Design review of the part built by this model. Coordinates are the model's own, in mm. A direction names the side the tool comes from. Coordinates: 2 decimals unless noted, no trailing zeros. Write each loop counter-clockwise with the first axis right and the second up, starting at its lowest first coordinate (ties: lowest second). Pieces come first, ordered by that corner, then holes. Notation, with made-up numbers: M -26,47 L 14,47 A15 cw 14,65 Z; hole C -9,-20.5 d8. An arc over 180 degrees is marked long. One line per question, with ' | ' between items.
from build123d import *

# Parameters (mm, degrees)
F0_W     = 50
F0_H     = 32
F0_R     = 1.25
F0_W_2   = 15
F0_H_2   = 4.5
F1_DEPTH = 10
F2_SIZE  = 5


with BuildPart() as f1:
    # F0 (on Top) → F1 (new body)
    with BuildSketch(Plane.XY):
        with Locations((25, 16)):
            Rectangle(F0_W, F0_H)
        with Locations((20, 4.85)):
            Circle(F0_R, mode=Mode.SUBTRACT)
        with Locations((30, 4.85)):
            Circle(F0_R, mode=Mode.SUBTRACT)
        with Locations((10, 16)):
            Rectangle(F0_W_2, F0_H_2, mode=Mode.SUBTRACT)
        with Locations((20, 27.15)):
            Circle(F0_R, mode=Mode.SUBTRACT)
        with Locations((40, 16)):
            Rectangle(F0_W_2, F0_H_2, mode=Mode.SUBTRACT)
        with Locations((30, 27.15)):
            Circle(F0_R, mode=Mode.SUBTRACT)
    extrude(amount=F1_DEPTH)

    # F2
    f2_edges = [f1.edges().sort_by_distance(p)[0] for p in [
        (0, 0, 5),
        (50, 0, 5),
        (50, 32, 5),
        (0, 32, 5),
    ]]
    chamfer(f2_edges, length=F2_SIZE)


solid = f1.part
1. Take a section at B-B (x = 30). Write out the cut boundary in (y, z).
Answer sheet:
outline: M 0,0 L 3.6,0 L 3.6,10 L 0,10 Z; M 6.1,0 L 25.9,0 L 25.9,10 L 6.1,10 Z; M 28.4,0 L 32,0 L 32,10 L 28.4,10 Z
2. To check wall thickness, follow line 1 along Y through (x, z) = (20, 5.25); line 2 along X through (y, z) = (17.5, 3); line 3 along Y through (x, z) = (5, 6.75). State the ranges of each line that lie inside material, in increasing order. Write a range as [from, to].
Answer sheet:
line 1: [0, 3.6], [6.1, 25.9], [28.4, 32] | line 2: [0, 2.5], [17.5, 32.5], [47.5, 50] | line 3: [0, 13.75], [18.25, 32]
3. Tool access review of faces 5 (the face through (17.5, 16, 5)), 6 (the face through (48, 29, 5)): name each direction out of +Z, -Z, +X, -X, +Y, -Y from which nothing blocks a thin tool from reaching the whole face with its end or side.
Answer sheet:
face 5: +Z, -Z | face 6: +Z, -Z, +X, +Y
4. Insertion check: pin 1 Ø1.5 at (x, y) = (30, 27.15) entering from -Z; pin 2 Ø3 at (x, y) = (15, 15) entering from +Z. Each pin has a flat end and moves straight along its axis. Give the tip position at first contact, or say it passes through.
Answer sheet:
pin 1: through | pin 2: z = 10
5. Take a section at A-A (z = 6.75). Write out the cut boundary in (x, y).
Answer sheet:
outline: M 0,5 L 5,0 L 45,0 L 50,5 L 50,27 L 45,32 L 5,32 L 0,27 Z; hole M 2.5,13.75 L 17.5,13.75 L 17.5,18.25 L 2.5,18.25 Z; hole C 20,4.85 d2.5; hole C 20,27.15 d2.5; hole C 30,4.85 d2.5; hole C 30,27.15 d2.5; hole M 32.5,13.75 L 47.5,13.75 L 47.5,18.25 L 32.5,18.25 Z
6. Draft analysis for pull direction Y (two halves, no side actions). For faces 1 (the face through (0, 16, 5)), 2 (the face through (10, 13.75, 5)), 3 (the face through (3, 2, 5)), 4 (the face through (30.672, 28.204, 4.93)), state which applies: pulls with the +Y half, pulls with the -Y half, needs draft (parallel to the pull), parting line crosses it, or undercut.
Answer sheet:
face 1: needs draft | face 2: undercut | face 3: pulls with the -Y half | face 4: undercut
